Here's how the part is built. I have some questions about the finished solid (model axes, mm). Face numbers are marked on the shaded views. A direction names the side the tool comes from. Coordinates: 2 decimals unless noted, no trailing zeros. Write each loop counter-clockwise with the first axis right and the second up, starting at its lowest first coordinate (ties: lowest second). Pieces come first, ordered by that corner, then holes.
(1) Please list where these lines run through material, in increasing order: probe 1 along Y at (x, z) = (-16.75, -4.75); probe 2 along Y at (x, z) = (-15.5, 3); probe 3 along Z at (x, y) = (-33, 13.5).
(2) Imagine slicing it at A-A, the plane z = -0.75. List the corners of the cut face in (x, y) for me, plus the area to 3 significant figures.
(3) Imagine slicing it at C-C, the plane y = -4. List the corners of the cut face in (x, z) for me.
(4) Which directions (+Z, -Z, +X, -X, +Y, -Y) give clear straight access to the entire face, cutting with the end or side of a thin tool? Please do the marked faces 1, 2 and 3.
(5) For pin 1 Ø1 at (y, z) = (-3, -6.5) entering from +X; pin 2 Ø5 at (x, z) = (-20, -2) entering from -Y, each with a flat end and sliding along its axis, tell me the tip position at first contact or that it passes through.
(6) Imagine slicing it at B-B, the plane z = -4.5. List the corners of the cut face in (x, y) for me, plus the area to 3 significant figures.
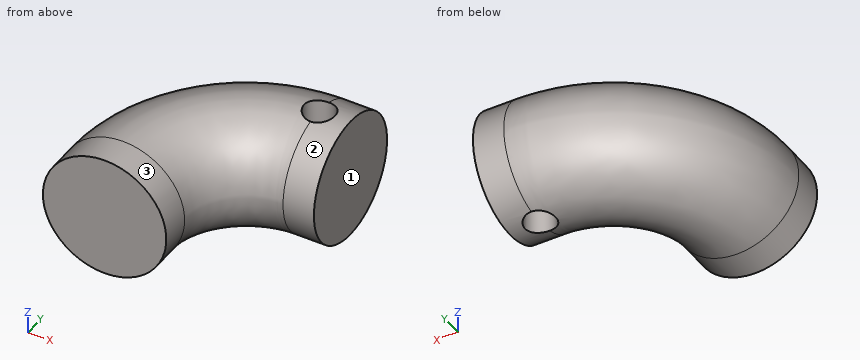
```python
from build123d import *

# Parameters (mm, degrees)
SWEEP_2_PROFILE_R        = 8
SKETCH_19_R              = 2
CUT_EXTRUDE_3_DEPTH      = 10
CUT_EXTRUDE_3_DEPTH_BACK = 10


with BuildPart() as part:
    # Sweep 2: sweep along a path in Sketch 1
    with BuildLine(Plane.XY) as sweep_2_path:
        Line((-32.264627437, -7.100709513), (-32.264627437, -3.100709513))
        ThreePointArc((-32.264627437, -3.100709513), (-27.578335936, 8.212998986), (-16.264627437, 12.899290487))
        Line((-16.264627437, 12.899290487), (-12.264627437, 12.899290487))
    # Sweep 2 profile (on start of the path) → Sweep 2 (sweep)
    with BuildSketch(Plane(origin=(-32.264627437, -7.100709513, 0), x_dir=(0, 0, 1), z_dir=(0, 1, 0))):
        Circle(SWEEP_2_PROFILE_R)
    sweep(path=sweep_2_path.line)

    # Sketch 19 → Cut-Extrude 3 (cut, two sides)
    with BuildSketch(Plane.XY) as cut_extrude_3_sk:
        with Locations((-16.264627437, 12.899290487)):
            Circle(SKETCH_19_R)
    extrude(amount=CUT_EXTRUDE_3_DEPTH, mode=Mode.SUBTRACT)
    extrude(cut_extrude_3_sk.sketch, amount=-CUT_EXTRUDE_3_DEPTH_BACK, mode=Mode.SUBTRACT)


solid = part.part
```
Recorded:
1. probe 1: y = 6.45 to 10.96, 14.84 to 19.33
1. probe 2: y = 5.48 to 11.05, 14.75 to 20.32
1. probe 3: z = -2.58 to 2.58
2. outline: (-40.23, -7.1) - (-24.3, -7.1) - (-24.3, -3.1) arc R8.04 cw to (-16.26, 4.93) - (-12.26, 4.93) - (-12.26, 20.86) - (-16.26, 20.86) arc R23.96 ccw to (-40.23, -3.1) - close; hole circle Ø4 at (-16.26, 12.9)
2. area: 515 mm2
3. outline: circle Ø16 at (-32.26, 0)
4. face 1: +Z, -Z, +X, +Y, -Y
4. face 2: +X
4. face 3: -Y
5. pin 1: stops at x = -26.97
5. pin 2: stops at y = 2.19
6. outline: (-38.88, -7.1) - (-25.65, -7.1) - (-25.65, -3.1) arc R9.39 cw to (-16.26, 6.28) - (-12.26, 6.28) - (-12.26, 19.51) - (-16.26, 19.51) arc R22.61 ccw to (-38.88, -3.1) - close; hole circle Ø4 at (-16.26, 12.9)
6. area: 426 mm2
